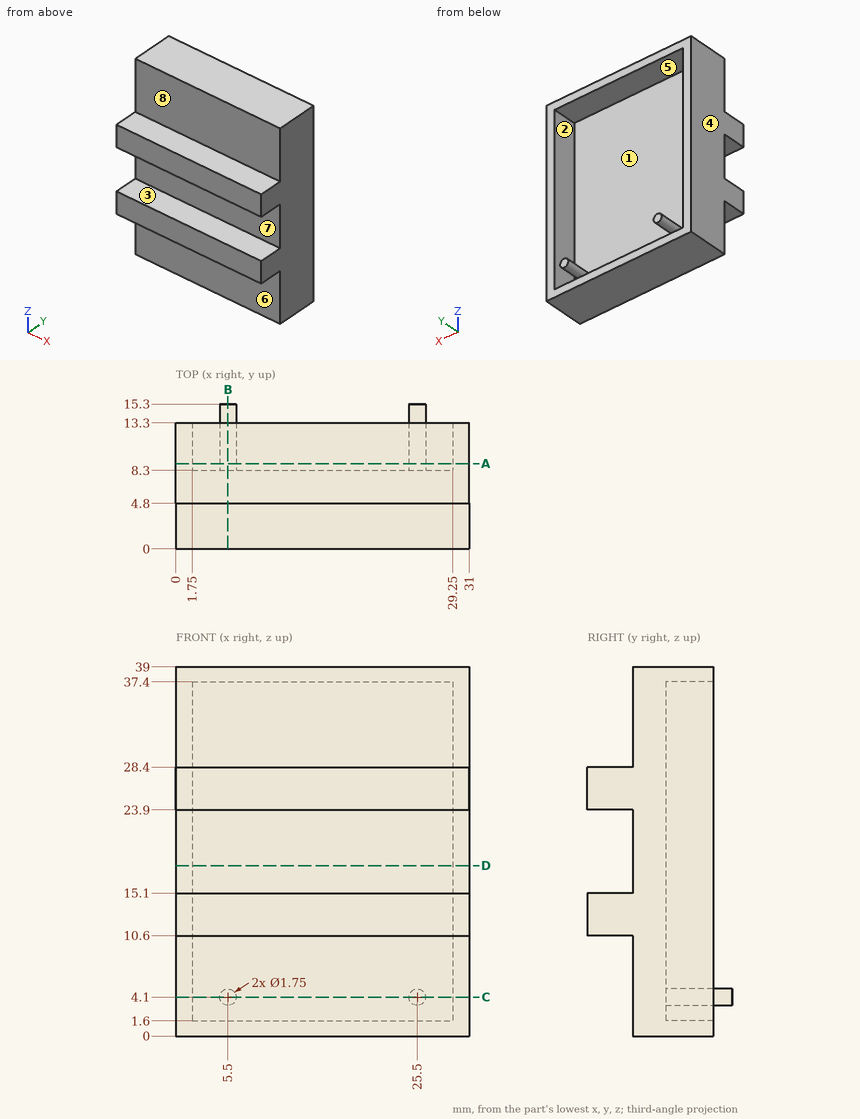
Study the drawing (mm; zero at the part's minimum x, y, z) and answer. A direction names the side the tool comes from. Round coordinates to 2 decimals unless told otherwise and drop trailing zeros. Write each loop counter-clockwise with the first axis right and the second up, starting at its lowest first coordinate (ties: lowest second). Pieces come first, ordered by that corner, then holes.
1) The mould has two halves that part along X. Classify the marked faces 1, 2, 3 and 4: pulls with the +X half, pulls with the -X half, needs draft (parallel to the pull), parting line crosses it, or undercut.
2) A cutting plane is placed at B-B (x = 5.5). Give the vertices of the cut face in (y, z) (3 decimals), plus the area to 3 significant figures.
3) Straight lines are drawn through the part: line 1 (Z direction, x = 11, y = 11); line 2 (X direction, y = 12.5, z = 12); line 3 (Z direction, x = 16, y = 3). For each, find the intervals that lie inside material, in ascending order.
4) A cutting plane is placed at A-A (y = 9). Give the vertices of the cut face in (x, z) (3 decimals).
5) A cutting plane is placed at C-C (z = 4.1). Give the vertices of the cut face in (x, y) (3 decimals), plus the area to 4 significant figures.
6) A tool of negligible diameter and unlimited length cuts with its end or side. For the marked faces 5, 6, 7 and 8, from which of +Z, -Z, +X, -X, +Y, -Y can it reach the whole face along a straight path? Write none if from no direction.
7) A cutting plane is placed at D-D (z = 18). Give the vertices of the cut face in (x, y), plus the area to 3 significant figures.
8) Given pin 1 Ø10 at (x, z) = (27, 11.5) entering from +Y; pin 2 Ø2.5 at (x, y) = (20.5, 2) entering from +Z; pin 3 Ø1.5 at (x, z) = (13.5, 31.5) entering from +Y, each flat-ended and moving along its own axis, determine where each tip first touches the part or whether it passes through.
Completed:
1. face 1: undercut
1. face 2: undercut
1. face 3: needs draft
1. face 4: pulls with the -X half
2. outline: (0, 10.6) - (4.8, 10.6) - (4.8, 0) - (13.3, 0) - (13.3, 1.6) - (8.3, 1.6) - (8.3, 3.225) - (15.3, 3.225) - (15.3, 4.975) - (8.3, 4.975) - (8.3, 37.4) - (13.3, 37.4) - (13.3, 39) - (4.8, 39) - (4.8, 28.4) - (0, 28.4) - (0, 23.9) - (4.8, 23.9) - (4.8, 15.1) - (0, 15.1) - close
2. area: 208 mm2
3. line 1: z = 0 to 1.6, 37.4 to 39
3. line 2: x = 0 to 1.75, 29.25 to 31
3. line 3: z = 10.6 to 15.1, 23.9 to 28.4
4. outline: (0, 0) - (31, 0) - (31, 39) - (0, 39) - close; circle Ø1.75 at (5.5, 4.1); circle Ø1.75 at (25.5, 4.1); hole (1.75, 1.6) - (29.25, 1.6) - (29.25, 37.4) - (1.75, 37.4) - close
5. outline: (0, 4.8) - (31, 4.8) - (31, 13.3) - (29.25, 13.3) - (29.25, 8.3) - (26.375, 8.3) - (26.375, 15.3) - (24.625, 15.3) - (24.625, 8.3) - (6.375, 8.3) - (6.375, 15.3) - (4.625, 15.3) - (4.625, 8.3) - (1.75, 8.3) - (1.75, 13.3) - (0, 13.3) - close
5. area: 150.5 mm2
6. face 5: +Y
6. face 6: -Z, +X, -X, -Y
6. face 7: +X, -X, -Y
6. face 8: +Z, +X, -X, -Y
7. outline: (0, 4.8) - (31, 4.8) - (31, 13.3) - (29.25, 13.3) - (29.25, 8.3) - (1.75, 8.3) - (1.75, 13.3) - (0, 13.3) - close
7. area: 126 mm2
8. pin 1: stops at y = 13.3
8. pin 2: stops at z = 28.4
8. pin 3: stops at y = 8.3
